from build123d import *

# Parameters (mm, degrees)
SKETCH1_R           = 10
BOSS_EXTRUDE1_DEPTH = 7.5


with BuildPart() as part:
    # Sketch1 → Boss-Extrude1 (new body)
    with BuildSketch(Plane(origin=(0, 0, 0), x_dir=(1, 0, 0), z_dir=(0, 1, 0))):
        with BuildLine():
            Line((14, 0), (14, 60))
            ThreePointArc((14, 60), (0, 74), (-14, 60))
            Line((-14, 60), (-14, 0))
            ThreePointArc((-14, 0), (0, -14), (14, 0))
        make_face()
        with BuildLine():
            ThreePointArc((4, 9.16515139), (0, -10), (-4, 9.16515139))
            Line((-4, 9.16515139), (-4, 5))
            Line((-4, 5), (4, 5))
            Line((4, 5), (4, 9.16515139))
        make_face(mode=Mode.SUBTRACT)
        with Locations((0, 60)):
            Circle(SKETCH1_R, mode=Mode.SUBTRACT)
    extrude(amount=BOSS_EXTRUDE1_DEPTH)


solid = part.part
Build history of the part. All positions in model axes, mm. A direction names the side the tool comes from. Coordinates: 2 decimals unless noted, no trailing zeros. Order: outer loops, then holes, each group sorted by start corner. A loop starts at its lowest first (then second) coordinate and runs counter-clockwise, first axis right, second up. Notation, with made-up numbers: (-13.5, 17.5) - (-4.5, 17.5) arc R21 cw to (-4.5, 23.5) - close; hole circle Ø3 at (37, -36). An arc over 180 degrees is marked (long way). Write each question's results on one line, items separated by ' | '. Start each with the question number.
Item 1: Flat gauge pins, fed straight in: pin 1 (4 mm diameter, centred on x = 7, y = 6, fed in from -Z); pin 2 (3 mm diameter, centred on x = 6.5, y = 1, fed in from +Z); pin 3 (3 mm diameter, centred on x = -6, y = 4, fed in from +Z). Where does each tip first touch, or does it go through?
Item 2: Band-saw the part on A-A on x = 0. Write the cut outline in (y, z), and give its area (4 significant figures).
Item 3: Tool access for faces 5 (the face through (4, 4, -7)), 6 (the face through (14, 4, -30)): list every direction of +Z, -Z, +X, -X, +Y, -Y with a clear straight run to the whole face (end or side of a thin tool).
Item 4: Mould opens along Z. For faces 1 (the face through (0, 4, -5)), 2 (the face through (0, 4, -74)), 3 (the face through (0, 7.5, -31)), 4 (the face through (0, 4, 14)) say: released by +Z, released by -Z, zero draft, split by the parting line, or undercut.
Item 5: Band-saw the part on B-B on y = 4.25. Write the cut outline in (x, z).
Item 6: Band-saw the part on C-C on z = -4. Write the cut outline in (x, y), and give its area (3 significant figures).
Item 7: Wall check: probe 1 along Z at (x, y) = (0, 5); probe 2 along X at (y, z) = (1, 0.5); probe 3 along Z at (x, y) = (-1.5, 1.25). Give the ranges that are in metal, low to high. Write a range as [from, to].
Item 8: Band-saw the part on D-D on z = 7.5. Write the cut outline in (x, y).
Numbers:
1) pin 1: z = -73.08 | pin 2: z = 13.08 | pin 3: z = 13.26
2) outline: (0, -74) - (7.5, -74) - (7.5, -70) - (0, -70) - close; (0, -50) - (7.5, -50) - (7.5, -5) - (0, -5) - close; (0, 10) - (7.5, 10) - (7.5, 14) - (0, 14) - close | area: 397.5 mm^2
3) face 5: +Y, -Y | face 6: +Z, -Z, +X, +Y, -Y
4) face 1: undercut | face 2: released by -Z | face 3: zero draft | face 4: released by +Z
5) outline: (-14, -60) arc R14 ccw to (14, -60) - (14, 0) arc R14 ccw to (-14, 0) - close; hole circle Ø20 at (0, -60); hole (-4, -9.17) - (-4, -5) - (4, -5) - (4, -9.17) arc R10 ccw (long way) to start
6) outline: (-14, 0) - (-9.17, 0) - (-9.17, 7.5) - (-14, 7.5) - close; (9.17, 0) - (14, 0) - (14, 7.5) - (9.17, 7.5) - close | area: 72.5 mm^2
7) probe 1: [-74, -70], [-50, -5], [10, 14] | probe 2: [-13.99, -9.99], [9.99, 13.99] | probe 3: [-73.92, -69.89], [-50.11, -5], [9.89, 13.92]
8) outline: (-11.82, 0) - (-6.61, 0) - (-6.61, 7.5) - (-11.82, 7.5) - close; (6.61, 0) - (11.82, 0) - (11.82, 7.5) - (6.61, 7.5) - close
